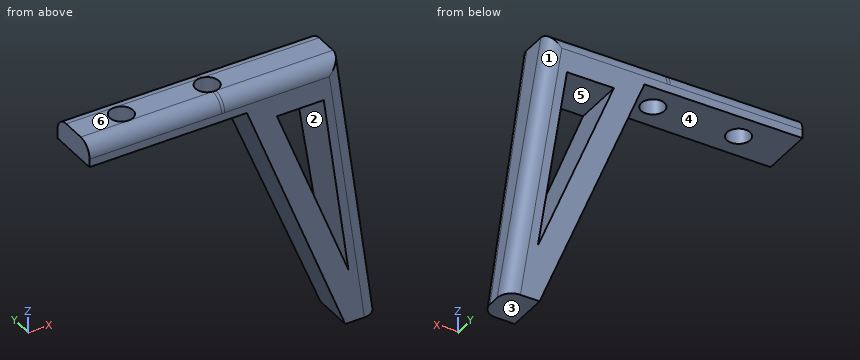
```python
from build123d import *

# Parameters (mm, degrees)
F1_DEPTH      = 11.5
F1_DEPTH_BACK = 7.25
F4_DEPTH      = 57.75
F5_R          = 2.032
F6_DEPTH      = 25
F7_R          = 2.5


# Not quite as in the source:
# - a feature names something its author has since deleted; it is built from what else it names


with BuildPart() as f1:
    # F0 (on Front) → F1 (new body, two sides)
    with BuildSketch(Plane.XZ) as f1_sk:
        Polygon((-26.8014297359, 2.0000000475), (-26.8014297359, -2.0000000475), (0.7941166829, -2.0000000475), (18.5593261492, -46.7420644607), (24.4487996128, -46.7420644607), (17.3888709152, 2.0000000475), align=None)
        Polygon((18.9966002603, -37.0041966029), (6.0891124744, -4.4964093445), (14.2880869367, -4.4964093445), align=None, mode=Mode.SUBTRACT)
    extrude(amount=F1_DEPTH)
    extrude(f1_sk.sketch, amount=-F1_DEPTH_BACK)

    # F3 (on offset) → F4 (cut)
    with BuildSketch(Plane(origin=(18.7998007554, 0, 2.7230125396), x_dir=(0, 1, 0), z_dir=(0.9896725236, 0, 0.1433467688))):
        Polygon((-18.5980091819, 10.2755831857), (-17.1822748397, -51.6943840463), (-3.4891957167, -51.8214939905), (-4.7216577223, 10.5497811385), align=None)
        Polygon((3.4891957167, -51.8214939905), (17.1822748397, -51.6943840463), (18.5980091819, 10.2755831857), (4.7216577223, 10.5497811385), align=None)
    extrude(amount=-F4_DEPTH, mode=Mode.SUBTRACT)

    # F5 (on face) → F6 (cut)
    with BuildSketch(Plane.XY.offset(2.0000000475)):
        with Locations((-3.4189070485, 0)):
            Circle(F5_R)
        with Locations((-18.4189070485, 0)):
            Circle(F5_R)
    extrude(amount=-F6_DEPTH, mode=Mode.SUBTRACT)

    # F7
    f7_edges = [f1.edges().sort_by_distance(p)[0] for p in [
        (-4.706279, -4.565636, 2),
        (-4.706279, 4.565636, 2),
        (20.918835, 4.016451, -22.371032),
        (20.918835, -4.016451, -22.371032),
    ]]
    fillet(f7_edges, radius=F7_R)


solid = f1.part
```
Could you check a few things on this model? Use its own coordinates, in mm. Face numbers are marked on the shaded views. A direction names the side the tool comes from. Round coordinates to 2 decimals unless told otherwise and drop trailing zeros. Loops run counter-clockwise (first coordinate to the right, second up) from the corner with the lowest first, then second, coordinate; pieces in that order, holes last. Notation, with made-up numbers: (28.25, 46) - (73.25, 46) arc R22 cw to (73.25, 78) - close; hole circle Ø6 at (19.5, -36). An arc over 180 degrees is marked (long way). Answer in a Markdown table with one row per item. Add a question column.
(1) I'm going to push flat-ended pins straight in: pin 1 (5 mm diameter, centred on y = -3.5, z = -6, fed in from -X); pin 2 (8 mm diameter, centred on x = -13.5, z = -4, fed in from -Y); pin 3 (1 mm diameter, centred on x = -2.5, y = -2.5, fed in from -Z). Where does each tip first touch, or does it pass through?
(2) I need wall thicknesses on line 1 along X through (y, z) = (-2, -32); line 2 along X through (y, z) = (-0.75, -27); line 3 along Z through (x, y) = (-20, 2.5). Which ranges of each line are inside material? Lowest first, please.
(3) For the marked faces 4, 5 and 6, which set-ups out of +Z, -Z, +X, -X, +Y, -Y let a thin tool reach every point of the face, with its end or its side?
(4) If we mould it in two halves opening along X, with no side actions, what happens to the marked faces 1, 2 and 3? For each: pulls with the +X half, pulls with the -X half, needs draft (parallel to the pull), parting line crosses it, or undercut.
(5) If we section it at A-A (y = 0): Please give me the cut outline in (x, z).
Model answer:
| question | item | result |
|---|---|---|
| 1 | pin 1 | stops at x = 1.39 |
| 1 | pin 2 | stops at y = -4.55 |
| 1 | pin 3 | stops at z = -2 |
| 2 | line 1 | x = 12.71 to 17.01, 18.27 to 22.22 |
| 2 | line 2 | x = 10.72 to 15.02, 17.55 to 21.59 |
| 2 | line 3 | z = -2 to 1.96 |
| 3 | face 4 | -Z, -X, +Y, -Y |
| 3 | face 5 | +Y, -Y |
| 3 | face 6 | +Z, +X, -X, +Y, -Y |
| 4 | face 1 | pulls with the +X half |
| 4 | face 2 | undercut |
| 4 | face 3 | needs draft |
| 5 | outline | (-26.8, -2) - (-20.45, -2) - (-20.45, 2) - (-26.8, 2) - close; (-16.39, -2) - (-5.45, -2) - (-5.45, 2) - (-16.39, 2) - close; (-1.39, -2) - (0.79, -2) - (18.56, -46.74) - (24.45, -46.74) - (17.39, 2) - (-1.39, 2) - close; hole (6.09, -4.5) - (19, -37) - (14.29, -4.5) - close |
